```python
from build123d import *

# Parameters (mm, degrees)
ESQUISSE1_R        = 1.75
BOSS_EXTRU_1_DEPTH = 3
ESQUISSE2_R        = 36
BOSS_EXTRU_4_DEPTH = 0.5
ESQUISSE5_R        = 36
ESQUISSE5_R_2      = 35
BOSS_EXTRU_6_DEPTH = 68
ESQUISSE6_R        = 36
BOSS_EXTRU_7_DEPTH = 2
CONG_7_R           = 3
CONG_8_R           = 3
CONG_9_R           = 3
CONG_10_R          = 3
CONG_11_R          = 3
CONG_12_R          = 3
CONG_13_R          = 3
CONG_15_R          = 3
CONG_16_R          = 3
ESQUISSE7_R        = 36.000000001
BOSS_EXTRU_9_DEPTH = 2.5


with BuildPart() as part:
    # Esquisse1 → Boss.-Extru.1 (new body)
    with BuildSketch(Plane(origin=(0, 0, 0), x_dir=(1, 0, 0), z_dir=(0, 1, 0))):
        Polygon((0, 91.06), (0, 0), (40, 0), (40, -14), (84, -14), (84, 0), (92, 0), (92, 39.56), (115, 39.56), (115, 83.56), (92, 83.56), (92, 91.06), align=None)
        with Locations(Location((108, 46.56, 0), (0, 0, 270))):
            Circle(ESQUISSE1_R, mode=Mode.SUBTRACT)
        with Locations(Location((108, 76.56, 0), (0, 0, 270))):
            Circle(ESQUISSE1_R, mode=Mode.SUBTRACT)
        with Locations(Location((3.5, 88.06, 0), (0, 0, 270))):
            Circle(ESQUISSE1_R, mode=Mode.SUBTRACT)
        with Locations(Location((77, -7, 0), (0, 0, 270))):
            Circle(ESQUISSE1_R, mode=Mode.SUBTRACT)
        with Locations(Location((47, -7, 0), (0, 0, 270))):
            Circle(ESQUISSE1_R, mode=Mode.SUBTRACT)
        Polygon((11.27, 87.06), (88, 87.06), (88, 6), (4.5, 6), (4.5, 73.06), (11.27, 73.06), align=None, mode=Mode.SUBTRACT)
    extrude(amount=-BOSS_EXTRU_1_DEPTH)

    # Esquisse2 → Boss.-Extru.4 (add)
    with BuildSketch(Plane(origin=(0, 0, 0), x_dir=(1, 0, 0), z_dir=(0, 1, 0))):
        Polygon((11.27, 73.06), (4.5, 73.06), (4.5, 6), (88, 6), (88, 87.06), (11.27, 87.06), align=None)
        with Locations(Location((46.25, 46.53, 0), (0, 0, 270))):
            Circle(ESQUISSE2_R, mode=Mode.SUBTRACT)
    extrude(amount=-BOSS_EXTRU_4_DEPTH)

    # Esquisse5 → Boss.-Extru.6 (add)
    with BuildSketch(Plane(origin=(0, 0, 0), x_dir=(1, 0, 0), z_dir=(0, 1, 0))):
        with Locations(Location((46.25, 46.53, 0), (0, 0, 270))):
            Circle(ESQUISSE5_R)
        with Locations(Location((46.25, 46.53, 0), (0, 0, 270))):
            Circle(ESQUISSE5_R_2, mode=Mode.SUBTRACT)
    extrude(amount=-BOSS_EXTRU_6_DEPTH)

    # Esquisse6 → Boss.-Extru.7 (add)
    with BuildSketch(Plane.XZ.offset(68)):
        with Locations(Location((46.25, -46.53, 0), (0, 0, 270))):
            Circle(ESQUISSE6_R)
    extrude(amount=BOSS_EXTRU_7_DEPTH)

    # Congé7
    cong_7_edges = [part.edges().sort_by_distance(p)[0] for p in [
        (0, -1.5, -91.06),
    ]]
    fillet(cong_7_edges, radius=CONG_7_R)

    # Congé8
    cong_8_edges = [part.edges().sort_by_distance(p)[0] for p in [
        (40, -1.5, 14),
    ]]
    fillet(cong_8_edges, radius=CONG_8_R)

    # Congé9
    cong_9_edges = [part.edges().sort_by_distance(p)[0] for p in [
        (0, -1.5, 0),
    ]]
    fillet(cong_9_edges, radius=CONG_9_R)

    # Congé10
    cong_10_edges = [part.edges().sort_by_distance(p)[0] for p in [
        (92, -1.5, 0),
    ]]
    fillet(cong_10_edges, radius=CONG_10_R)

    # Congé11
    cong_11_edges = [part.edges().sort_by_distance(p)[0] for p in [
        (84, -1.5, 14),
    ]]
    fillet(cong_11_edges, radius=CONG_11_R)

    # Congé12
    cong_12_edges = [part.edges().sort_by_distance(p)[0] for p in [
        (115, -1.5, -39.56),
    ]]
    fillet(cong_12_edges, radius=CONG_12_R)

    # Congé13
    cong_13_edges = [part.edges().sort_by_distance(p)[0] for p in [
        (115, -1.5, -83.56),
    ]]
    fillet(cong_13_edges, radius=CONG_13_R)

    # Congé15
    cong_15_edges = [part.edges().sort_by_distance(p)[0] for p in [
        (92, -1.5, -91.06),
    ]]
    fillet(cong_15_edges, radius=CONG_15_R)

    # Congé16
    cong_16_edges = [part.edges().sort_by_distance(p)[0] for p in [
        (46.25, -70, -10.53),
    ]]
    fillet(cong_16_edges, radius=CONG_16_R)

    # Esquisse7 → Boss.-Extru.9 (add)
    with BuildSketch(Plane.XZ.offset(0.5)):
        Polygon((4.5, -6), (88, -6), (88, -87.06), (11.27, -87.06), (11.27, -73.06), (4.5, -73.06), align=None)
        with Locations(Location((46.25, -46.53, 0), (0, 0, 270))):
            Circle(ESQUISSE7_R, mode=Mode.SUBTRACT)
    extrude(amount=BOSS_EXTRU_9_DEPTH)


solid = part.part
```
The listing builds one solid part. Answer for the finished solid, in the listing's coordinates (mm). A direction names the side the tool comes from. Coordinates: 2 decimals unless noted, no trailing zeros. Write each loop counter-clockwise with the first axis right and the second up, starting at its lowest first coordinate (ties: lowest second). Pieces come first, ordered by that corner, then holes. Notation, with made-up numbers: (52.25, 86) - (86.25, 86) arc R23 cw to (86.25, 98) - close; hole circle Ø8 at (26, 50.5). An arc over 180 degrees is marked (long way). Return JSON: item names as keys, results as strings. Group by question number.
Q1. Flat-ended cylindrical pins translate along their axes: pin 1 Ø2.5 at (x, y) = (104, -1.5) entering from +Z; pin 2 Ø2.5 at (y, z) = (-2, -86) entering from +X; pin 3 Ø1 at (x, y) = (13.5, -28.5) entering from -Z. Find the tip coordinate at first contact, or state that the pin passes through.
Q2. Which of the six approach directions +Z, -Z, +X, -X, +Y, -Y give full straight-line access (tool end or side, diameter ignored) to faces 4 (the flat face through (92, -1, -21)), 5 (the flat face through (92, -1, -86)), 6 (the flat face through (47, -70, -46)), 7 (the cylindrical face through (11.1, -34.6, -54.3)), 8 (the flat face through (47, -68, -46))?
Q3. Find the intervals of material crossed by line 1 along Z through (x, y) = (108, -1.3); line 2 along X through (y, z) = (-2.2, 7); line 3 along Z through (x, y) = (77, -0.6), in increasing order. Write a range as [from, to].
Q4. The part is cut by section B-B on y = -10.5. Write down the section's boundary in (x, z).
Q5. For a pull along X with two mould halves and no side action, classify faces 1 (the flat face through (102, -1, -83.56)), 2 (the cylindrical face through (80.95, -33.52, -51.09)), 3 (the flat face through (0, -1, -46)) as +X half, -X half, draft (parallel to the pull), parting line (faces both ways), or undercut.
Q6. The part is cut by section A-A on z = 7. Write down the section's boundary in (x, y).
Evaluation:
{
 "1": {"pin 1": "stops at z = -39.56", "pin 2": "stops at x = 92", "pin 3": "stops at z = -62.53"},
 "2": {"face 4": "+Z, +X, +Y, -Y", "face 5": "-Z, +X, +Y, -Y", "face 6": "+Z, -Z, +X, -X, -Y", "face 7": "-Y", "face 8": "+Y"},
 "3": {"line 1": "z = [-83.56, -78.31], [-74.81, -48.31], [-44.81, -39.56]", "line 2": "x = [40, 45.25], [48.75, 75.25], [78.75, 84]", "line 3": "z = [-91.06, -63.25], [-29.81, 5.25], [8.75, 14]"},
 "4": {"outline": "circle Ø72 at (46.25, -46.53); hole circle Ø70 at (46.25, -46.53)"},
 "5": {"face 1": "draft", "face 2": "undercut", "face 3": "-X half"},
 "6": {"outline": "(40, -3) - (45.25, -3) - (45.25, 0) - (40, 0) - close; (48.75, -3) - (75.25, -3) - (75.25, 0) - (48.75, 0) - close; (78.75, -3) - (84, -3) - (84, 0) - (78.75, 0) - close"}
}
